Build history of the part. All positions in model axes, mm. Face numbers are marked on the shaded views. A direction names the side the tool comes from. Round coordinates to 2 decimals unless told otherwise and drop trailing zeros. Order: outer loops, then holes, each group sorted by start corner. A loop starts at its lowest first (then second) coordinate and runs counter-clockwise, first axis right, second up. Notation, with made-up numbers: M 34,-40 L 66,-40 A14 cw 66,-15 Z; hole C 60.25,4.5 d6. An arc over 180 degrees is marked long. One line per item, written item: value. Start each with the question number.
Item 1: Two-plate mould, pull along Z, no slides. Class the marked faces 1, 2 and 3: +Z half, -Z half, draft (parallel to the pull), parting line (faces both ways), or undercut.
Item 2: Pin check, flat tips, straight feed: pin 1 (23.5 mm diameter, centred on y = -10, z = 1, fed in from +X); pin 2 (4 mm diameter, centred on x = 98, y = 2.5, fed in from +Z); pin 3 (3 mm diameter, centred on x = 117.5, y = 23, fed in from -Z). Stop position of each tip, or through.
Item 3: Probe L1, parallel to X at y = 32, z = 12; L2, parallel to Y at x = 146.5, z = 0; L3, parallel to Z at x = 38, y = 14.5. List the from-to ranges inside material, lowest first.
Item 4: Tool access for the marked faces 4, 5 and 6: list every direction of +Z, -Z, +X, -X, +Y, -Y with a clear straight run to the whole face (end or side of a thin tool).
Item 5: Band-saw the part on A-A, the plane x = 46. Write the cut outline in (y, z).
```python
from build123d import *

# Parameters (mm, degrees)
SKETCH1_R            = 15
BOSS_EXTRUDE1_DEPTH  = 5.5
SKETCH2_R            = 23.5
BOSS_EXTRUDE2_DEPTH  = 12
SKETCH4_R            = 19.5
BOSS_EXTRUDE3_DEPTH  = 11.8
SKETCH6_R            = 20.25
BOSS_EXTRUDE4_DEPTH  = 6.7
SKETCH7_R            = 35.15
BOSS_EXTRUDE5_DEPTH  = 6
SKETCH8_R            = 33.5
BOSS_EXTRUDE6_DEPTH  = 8
SKETCH9_R            = 32
BOSS_EXTRUDE7_DEPTH  = 9
SKETCH10_R           = 35.15
BOSS_EXTRUDE8_DEPTH  = 7
SKETCH11_R           = 33.5
BOSS_EXTRUDE9_DEPTH  = 9
SKETCH12_R           = 32
BOSS_EXTRUDE10_DEPTH = 9
SKETCH13_R           = 34
BOSS_EXTRUDE11_DEPTH = 9
SKETCH14_R           = 35.15
BOSS_EXTRUDE12_DEPTH = 7
SKETCH15_R           = 35
BOSS_EXTRUDE13_DEPTH = 64


with BuildPart() as part:
    # Sketch1 → Boss-Extrude1 (new body)
    with BuildSketch(Plane(origin=(0, 0, 0), x_dir=(0, 0, -1), z_dir=(1, 0, 0))):
        Circle(SKETCH1_R)
    extrude(amount=BOSS_EXTRUDE1_DEPTH)

    # Sketch2 → Boss-Extrude2 (add)
    with BuildSketch(Plane(origin=(5.5, 0, 0), x_dir=(0, 0, -1), z_dir=(1, 0, 0))):
        Circle(SKETCH2_R)
    extrude(amount=BOSS_EXTRUDE2_DEPTH)

    # Sketch4 → Boss-Extrude3 (add)
    with BuildSketch(Plane(origin=(17.5, 0, 0), x_dir=(0, 0, -1), z_dir=(1, 0, 0))):
        Circle(SKETCH4_R)
    extrude(amount=BOSS_EXTRUDE3_DEPTH)

    # Sketch6 → Boss-Extrude4 (add)
    with BuildSketch(Plane(origin=(29.3, 0, 0), x_dir=(0, 0, -1), z_dir=(1, 0, 0))):
        Circle(SKETCH6_R)
    extrude(amount=BOSS_EXTRUDE4_DEPTH)

    # Sketch7 → Boss-Extrude5 (add)
    with BuildSketch(Plane(origin=(36, 0, 0), x_dir=(0, 0, -1), z_dir=(1, 0, 0))):
        Circle(SKETCH7_R)
    extrude(amount=BOSS_EXTRUDE5_DEPTH)

    # Sketch8 → Boss-Extrude6 (add)
    with BuildSketch(Plane(origin=(42, 0, 0), x_dir=(0, 0, -1), z_dir=(1, 0, 0))):
        Circle(SKETCH8_R)
    extrude(amount=BOSS_EXTRUDE6_DEPTH)

    # Sketch9 → Boss-Extrude7 (add)
    with BuildSketch(Plane(origin=(50, 0, 0), x_dir=(0, 0, -1), z_dir=(1, 0, 0))):
        Circle(SKETCH9_R)
    extrude(amount=BOSS_EXTRUDE7_DEPTH)

    # Sketch10 → Boss-Extrude8 (add)
    with BuildSketch(Plane(origin=(59, 0, 0), x_dir=(0, 0, -1), z_dir=(1, 0, 0))):
        Circle(SKETCH10_R)
    extrude(amount=BOSS_EXTRUDE8_DEPTH)

    # Sketch11 → Boss-Extrude9 (add)
    with BuildSketch(Plane(origin=(66, 0, 0), x_dir=(0, 0, -1), z_dir=(1, 0, 0))):
        Circle(SKETCH11_R)
    extrude(amount=BOSS_EXTRUDE9_DEPTH)

    # Sketch12 → Boss-Extrude10 (add)
    with BuildSketch(Plane(origin=(75, 0, 0), x_dir=(0, 0, -1), z_dir=(1, 0, 0))):
        Circle(SKETCH12_R)
    extrude(amount=BOSS_EXTRUDE10_DEPTH)

    # Sketch13 → Boss-Extrude11 (add)
    with BuildSketch(Plane(origin=(84, 0, 0), x_dir=(0, 0, -1), z_dir=(1, 0, 0))):
        Circle(SKETCH13_R)
    extrude(amount=BOSS_EXTRUDE11_DEPTH)

    # Sketch14 → Boss-Extrude12 (add)
    with BuildSketch(Plane(origin=(93, 0, 0), x_dir=(0, 0, -1), z_dir=(1, 0, 0))):
        Circle(SKETCH14_R)
    extrude(amount=BOSS_EXTRUDE12_DEPTH)

    # Sketch15 → Boss-Extrude13 (add)
    with BuildSketch(Plane(origin=(100, 0, 0), x_dir=(0, 0, -1), z_dir=(1, 0, 0))):
        Circle(SKETCH15_R)
    extrude(amount=BOSS_EXTRUDE13_DEPTH)

    # Sketch16 → Cut-Revolve1 (revolve, cut)
    with BuildSketch(Plane(origin=(0, 0, 0), x_dir=(1, 0, 0), z_dir=(0, 1, 0))):
        with BuildLine():
            Line((164, 30.145778452), (104.875699315, 30.145778452))
            add(Edge.make_bspline(
                [(104.875699315, 30.145778452), (111.575177395, 21.323772465), (113.598201805, 11.115911288), (113.598201805, 0)],
                knots=[0, 0, 0, 0, 1, 1, 1, 1], degree=3))
            Line((113.598201805, 0), (164, 0))
            Line((164, 0), (164, 30.145778452))
        make_face()
    revolve(axis=Axis((164, 0, 0), (-1, 0, 0)), mode=Mode.SUBTRACT)


solid = part.part
```
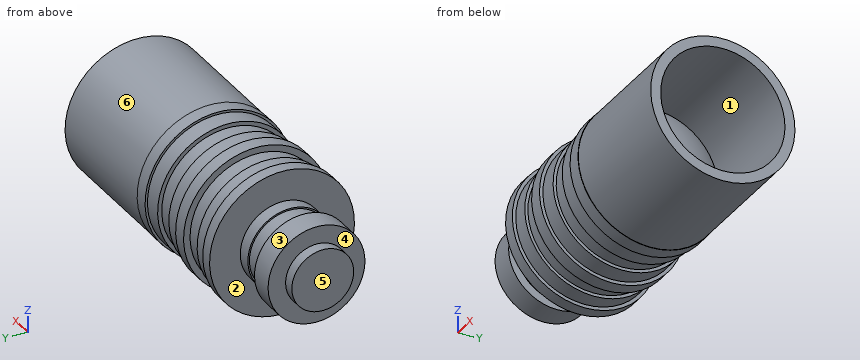
Output:
1. face 1: undercut
1. face 2: draft
1. face 3: parting line
2. pin 1: stops at x = 113.6
2. pin 2: stops at z = 35.15
2. pin 3: stops at z = -27.62
3. L1: x = 36 to 42, 59 to 66, 93 to 164
3. L2: y = -35 to -30.15, 30.15 to 35
3. L3: z = -32.02 to 32.02
4. face 4: -X
4. face 5: +Z, -Z, -X, +Y, -Y
4. face 6: +X
5. outline: C 0,0 d67
